```python
from build123d import *

# Parameters (mm, degrees)
SKETCH1_W           = 2.9972
SKETCH1_H           = 4.445
BOSS_EXTRUDE1_DEPTH = 2.9972


with BuildPart() as part:
    # Sketch1 → Boss-Extrude1 (new body)
    with BuildSketch(Plane.XY):
        Polygon((0, 19.2778), (0, 10.3878), (6.096, 10.3878), (6.096, 7.3398), (107.696, 7.3398), (107.696, 10.3878), (113.792, 10.3878), (113.792, 19.2778), (107.696, 19.2778), (6.096, 19.2778), align=None)
        with Locations((18.796, 12.6103)):
            Rectangle(SKETCH1_W, SKETCH1_H, mode=Mode.SUBTRACT)
        with Locations((37.846, 12.6103)):
            Rectangle(SKETCH1_W, SKETCH1_H, mode=Mode.SUBTRACT)
        with Locations((56.896, 12.6103)):
            Rectangle(SKETCH1_W, SKETCH1_H, mode=Mode.SUBTRACT)
        with Locations((75.946, 12.6103)):
            Rectangle(SKETCH1_W, SKETCH1_H, mode=Mode.SUBTRACT)
        with Locations((94.996, 12.6103)):
            Rectangle(SKETCH1_W, SKETCH1_H, mode=Mode.SUBTRACT)
    extrude(amount=BOSS_EXTRUDE1_DEPTH)


solid = part.part
```
Geometry check sheet. Reference: the model listing, model coordinates, mm. A direction names the side the tool comes from. Round coordinates to 2 decimals unless told otherwise and drop trailing zeros. Write each loop counter-clockwise with the first axis right and the second up, starting at its lowest first coordinate (ties: lowest second). Pieces come first, ordered by that corner, then holes. Notation, with made-up numbers: (11, -39) - (51, -39) arc R29 cw to (51, -13) - close; hole circle Ø1 at (44.5, 21). An arc over 180 degrees is marked (long way). Write each question's results on one line, items separated by ' | '.
(1) Depth check by flat-ended pin: pin 1 Ø0.9 at (x, z) = (109, 1) entering from -Y; pin 2 Ø0.9 at (y, z) = (9.5, 1.5) entering from +X. Enter the tip coordinate at first touch or a pass-through.
Computed:
pin 1: stops at y = 10.39 | pin 2: stops at x = 107.7
(2) Sectioned sample at B-B, the plane y = 11.5. Enter the section's corners in (x, z), plus the area to 3 significant figures.
Computed:
outline: (0, 0) - (17.3, 0) - (17.3, 3) - (0, 3) - close; (20.29, 0) - (36.35, 0) - (36.35, 3) - (20.29, 3) - close; (39.34, 0) - (55.4, 0) - (55.4, 3) - (39.34, 3) - close; (58.39, 0) - (74.45, 0) - (74.45, 3) - (58.39, 3) - close; (77.44, 0) - (93.5, 0) - (93.5, 3) - (77.44, 3) - close; (96.49, 0) - (113.79, 0) - (113.79, 3) - (96.49, 3) - close | area: 296 mm^2
(3) Set-up check for faces 1 (the face through (107.696, 9, 1)), 2 (the face through (55.397, 13, 1)), 3 (the face through (6.096, 9, 1)): record each of +Z, -Z, +X, -X, +Y, -Y from which the full face is reachable in a straight line by a thin tool's end or side.
Computed:
face 1: +Z, -Z, +X, -Y | face 2: +Z, -Z | face 3: +Z, -Z, -X, -Y
(4) Sectioned sample at A-A, the plane z = 1.85. Enter the section's corners in (x, y).
Computed:
outline: (0, 10.39) - (6.1, 10.39) - (6.1, 7.34) - (107.7, 7.34) - (107.7, 10.39) - (113.79, 10.39) - (113.79, 19.28) - (0, 19.28) - close; hole (17.3, 10.39) - (20.29, 10.39) - (20.29, 14.83) - (17.3, 14.83) - close; hole (36.35, 10.39) - (39.34, 10.39) - (39.34, 14.83) - (36.35, 14.83) - close; hole (55.4, 10.39) - (58.39, 10.39) - (58.39, 14.83) - (55.4, 14.83) - close; hole (74.45, 10.39) - (77.44, 10.39) - (77.44, 14.83) - (74.45, 14.83) - close; hole (93.5, 10.39) - (96.49, 10.39) - (96.49, 14.83) - (93.5, 14.83) - close
(5) Thickness scan on probe 1 along X at (y, z) = (12.5, 0.75); probe 2 along Y at (x, z) = (37, 2.7); probe 3 along X at (y, z) = (9, 0.6). Record the ranges inside material, lowest first. Write a range as from..to.
Computed:
probe 1: x = 0..17.3, 20.29..36.35, 39.34..55.4, 58.39..74.45, 77.44..93.5, 96.49..113.79 | probe 2: y = 7.34..10.39, 14.83..19.28 | probe 3: x = 6.1..107.7
(6) Draft check along Y on faces 4 (the face through (58, 19.278, 1)), 5 (the face through (56, 16, 0)), 6 (the face through (38, 10.388, 1)). Enter one of: pulls with the +Y half, pulls with the -Y half, needs draft (parallel to the pull), parting line crosses it, or undercut.
Computed:
face 4: pulls with the +Y half | face 5: needs draft | face 6: undercut
